```python
from build123d import *

# Parameters (mm, degrees)
BOSS_EXTRUDE1_DEPTH = 5
SKETCH4_R           = 0.175
CUT_EXTRUDE1_DEPTH  = 13.583057392


with BuildPart() as part:
    # Sketch1 → Boss-Extrude1 (new body)
    with BuildSketch(Plane(origin=(0, 0, 0), x_dir=(1, 0, 0), z_dir=(0, 1, 0))):
        Polygon((5.773502692, 0), (2.886751346, 5), (-2.886751346, 5), (-5.773502692, 0), (-2.886751346, -5), (2.886751346, -5), align=None)
    extrude(amount=-BOSS_EXTRUDE1_DEPTH)

    # Sketch3 → Revolve1 (revolve)
    with BuildSketch(Plane.XY):
        Polygon((0, -5), (0, -10), (-5, -5), align=None)
    revolve(axis=Axis((0, -5, 0), (0, -1, 0)))

    # Sketch4 → Cut-Extrude1 (cut, through all)
    with BuildSketch(Plane(origin=(0, 0, 0), x_dir=(1, 0, 0), z_dir=(0, 1, 0))):
        with Locations(Location((0, 0, 0), (0, 0, 270))):
            Circle(SKETCH4_R)
    extrude(amount=-CUT_EXTRUDE1_DEPTH, mode=Mode.SUBTRACT)


solid = part.part
```
Here's how the part is built. I have some questions about the finished solid (model axes, mm). A direction names the side the tool comes from. Round coordinates to 2 decimals unless told otherwise and drop trailing zeros. Write each loop counter-clockwise with the first axis right and the second up, starting at its lowest first coordinate (ties: lowest second). Pieces come first, ordered by that corner, then holes.
Q1. Will these pins go through, and if not, where does the flat tip stop? P1, Ø0.7, axis at x = 5, z = -1, coming from the -Y side; P2, Ø1.2, axis at x = -5, z = -1, coming from the -Y side; P3, Ø1.3, axis at x = -2, z = 3, coming from the -Y side.
Q2. If we section it at C-C on y = -8: Write out the boundary of the cut face in (x, z) (3 decimals).
Q3. Please list where these lines run through material, in increasing order: probe 1 along Z at (x, y) = (0, -3) (3 decimals); probe 2 along X at (y, z) = (-5.5, 0) (3 decimals); probe 3 along X at (y, z) = (-2.75, -4.5).
Q4. If we section it at B-B on y = -7: Write out the boundary of the cut face in (x, z) (3 decimals).
Q5. Which directions (+Z, -Z, +X, -X, +Y, -Y) give clear straight access to the entire face, cutting with the end or side of a thin tool? Please do faces 1 (the flat face through (2.6, -5, -4.5)), 2 (the flat face through (-2.7, -5, -4.5)), 3 (the flat face through (2.6, -5, 4.5)), 4 (the flat face through (5.2, -5, 0)), 5 (the flat face through (-2.7, -5, 4.5)).
Answer below:
1. P1: stops at y = -5.25
1. P2: stops at y = -5.5
1. P3: stops at y = -7.04
2. outline: circle Ø4 at (0, 0); hole circle Ø0.35 at (0, 0)
3. probe 1: z = -5 to -0.175, 0.175 to 5
3. probe 2: x = -4.5 to -0.175, 0.175 to 4.5
3. probe 3: x = -3.18 to 3.18
4. outline: circle Ø6 at (0, 0); hole circle Ø0.35 at (0, 0)
5. face 1: -Z, +X, -Y
5. face 2: -Z, -X, -Y
5. face 3: +Z, +X, -Y
5. face 4: +X, -Y
5. face 5: +Z, -X, -Y
